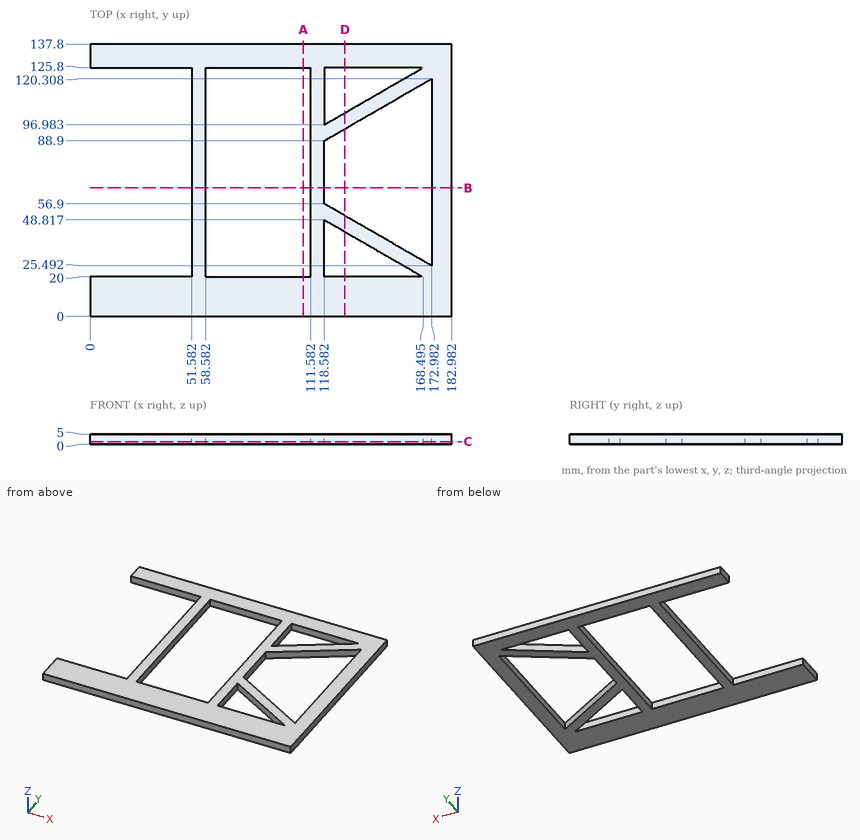
Design review of the part shown in the three views and the two pictorial views. Dimensions are in mm from the part's minimum x, y and z. Give positions to 0.01 mm unless a question says otherwise; leave off trailing zeros. Write each loop counter-clockwise with the first axis right and the second up, starting at its lowest first coordinate (ties: lowest second). Pieces come first, ordered by that corner, then holes.
(1) Add section C-C (z = 1.35). Give the boundary of the cut face in (x, y) (1 decimal).
Checked values:
outline: (0, 0) - (183, 0) - (183, 137.8) - (0, 137.8) - (0, 125.8) - (51.6, 125.8) - (51.6, 20) - (0, 20) - close; hole (58.6, 20) - (111.6, 20) - (111.6, 125.8) - (58.6, 125.8) - close; hole (118.6, 20) - (168.5, 20) - (118.6, 48.8) - close; hole (118.6, 56.9) - (173, 25.5) - (173, 120.3) - (118.6, 88.9) - close; hole (118.6, 97) - (168.5, 125.8) - (118.6, 125.8) - close
(2) Add section A-A (x = 108). Give the boundary of the cut face in (y, z).
Checked values:
outline: (0, 0) - (20, 0) - (20, 5) - (0, 5) - close; (125.8, 0) - (137.8, 0) - (137.8, 5) - (125.8, 5) - close
(3) Clearance check with flat-ended pins moving along their axes: pin 1 Ø1.5 at (y, z) = (52.5, 3) entering from -X; pin 2 Ø1.5 at (x, z) = (85, 3.5) entering from -Y. State where each tip first meets the part, or that it passes through.
Checked values:
pin 1: stops at x = 51.58
pin 2: stops at y = 0
(4) Add section B-B (y = 65). Give the boundary of the cut face in (x, z).
Checked values:
outline: (51.58, 0) - (58.58, 0) - (58.58, 5) - (51.58, 5) - close; (111.58, 0) - (118.58, 0) - (118.58, 5) - (111.58, 5) - close; (172.98, 0) - (182.98, 0) - (182.98, 5) - (172.98, 5) - close
(5) Wall thickness on line 1 along X through (y, z) = (87, 1.35); line 2 along Y through (x, z) = (102, 2.4); line 3 along X through (y, z) = (42, 0.35) (1 decimal): over which ranges is each line inside the solid? List them lowest first.
Checked values:
line 1: x = 51.58 to 58.58, 111.58 to 118.58, 172.98 to 182.98
line 2: y = 0 to 20, 125.8 to 137.8
line 3: x = 51.6 to 58.6, 111.6 to 118.6, 130.4 to 144.4, 173 to 183
(6) Add section D-D (x = 129). Give the boundary of the cut face in (y, z) (1 decimal).
Checked values:
outline: (0, 0) - (20, 0) - (20, 5) - (0, 5) - close; (42.8, 0) - (50.9, 0) - (50.9, 5) - (42.8, 5) - close; (94.9, 0) - (103, 0) - (103, 5) - (94.9, 5) - close; (125.8, 0) - (137.8, 0) - (137.8, 5) - (125.8, 5) - close
